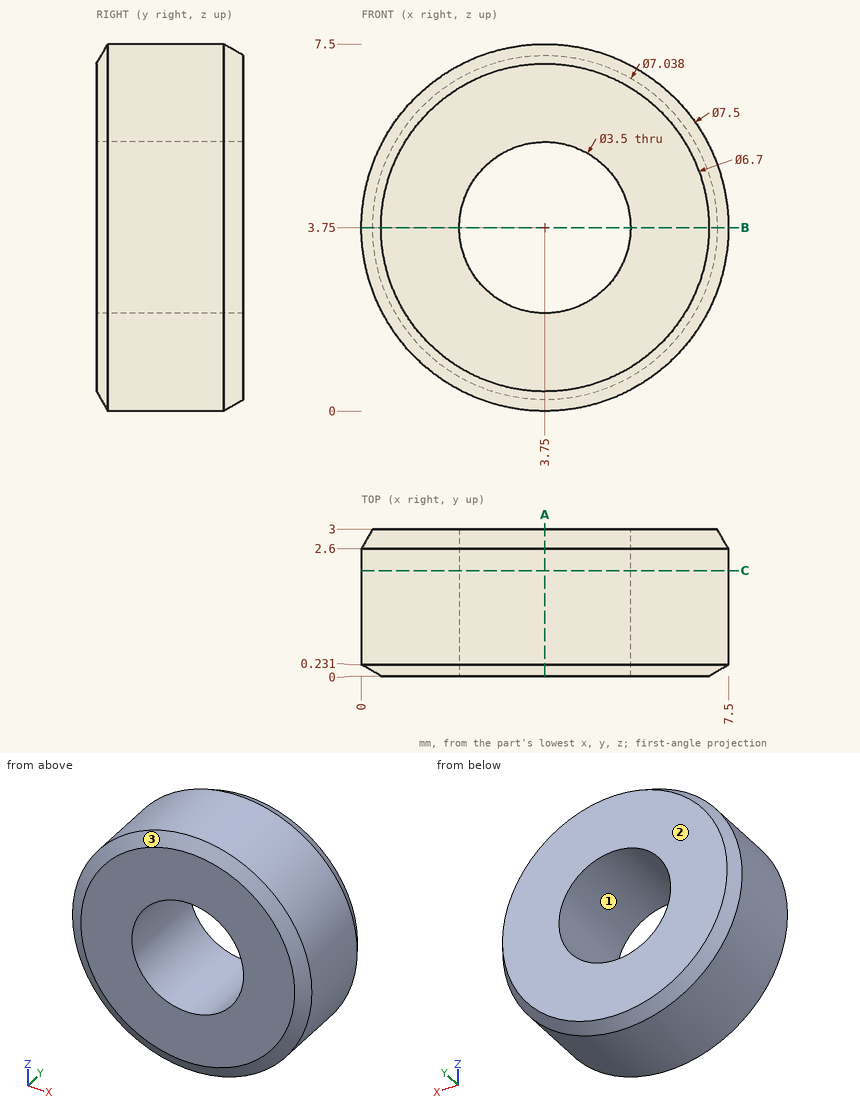
Design review of the part shown in the three views and the two pictorial views. Dimensions are in mm from the part's minimum x, y and z. Round coordinates to 2 decimals unless told otherwise and drop trailing zeros. Write each loop counter-clockwise with the first axis right and the second up, starting at its lowest first coordinate (ties: lowest second). Pieces come first, ordered by that corner, then holes. Notation, with made-up numbers: M 23.25,-32.75 L 74.25,-32.75 A25 cw 74.25,-2.75 Z; hole C -12,65 d5. An arc over 180 degrees is marked long. Use a Markdown table: item, result. Add a question column.
Q1. To check wall thickness, follow line 1 (X direction, y = 1.5, z = 3.75); line 2 (X direction, y = 0.5, z = 4.5). State the ranges of each line that lie inside material, in increasing order.
Q2. We need section A-A, the plane x = 3.75. State the section outline as (y, z) points, plus the area to 3 significant figures.
Q3. We need section B-B, the plane z = 3.75. State the section outline as (x, y) points.
Q4. We need section C-C, the plane y = 2.15. State the section outline as (x, z) points.
Q5. Insertion check: pin 1 (1.5 mm diameter, centred on y = 1, z = 5, fed in from +X); pin 2 (3 mm diameter, centred on x = 3.75, z = 3.75, fed in from -Y) (3 decimals). Each pin has a flat end and moves straight along its axis. Give the tip position at first contact, or say it passes through.
Q6. The part is to be moulded in two halves that separate along Z. For the marked faces 1, 2 and 3, say which applies: pulls with the +Z half, pulls with the -Z half, needs draft (parallel to the pull), parting line crosses it, or undercut.
Findings below:
| question | item | result |
|---|---|---|
| 1 | line 1 | x = 0 to 2, 5.5 to 7.5 |
| 1 | line 2 | x = 0.08 to 2.17, 5.33 to 7.42 |
| 2 | outline | M 0,0.4 L 0.23,0 L 2.6,0 L 3,0.23 L 3,2 L 0,2 Z; M 0,5.5 L 3,5.5 L 3,7.27 L 2.6,7.5 L 0.23,7.5 L 0,7.1 Z |
| 2 | area | 11.8 mm² |
| 3 | outline | M 0,0.23 L 0.4,0 L 2,0 L 2,3 L 0.23,3 L 0,2.6 Z; M 5.5,0 L 7.1,0 L 7.5,0.23 L 7.5,2.6 L 7.27,3 L 5.5,3 Z |
| 4 | outline | C 3.75,3.75 d7.5; hole C 3.75,3.75 d3.5 |
| 5 | pin 1 | stops at x = 7.47 |
| 5 | pin 2 | passes through |
| 6 | face 1 | undercut |
| 6 | face 2 | needs draft |
| 6 | face 3 | parting line crosses it |
